Input: part model. Units: mm. Frame: model coordinates. Give positions to 0.01 mm unless a question says otherwise; leave off trailing zeros. Write each loop counter-clockwise with the first axis right and the second up, starting at its lowest first coordinate (ties: lowest second). Pieces come first, ordered by that corner, then holes. Notation, with made-up numbers: (-31.5, 4) -> (-10.5, 4) arc R17 cw to (-10.5, 15) -> close; hole circle Ø10 at (73, -31.75). An arc over 180 degrees is marked (long way). Return JSON: item names as keys, results as strings. Group by question number.
Item 1: Section C-C, the plane z = 5. Count the separate pieces of the cut face and the enclosed holes in it, then the cut area to 3 significant figures.
Item 2: Section A-A, the plane y = 0. Return loops of the section in (x, z), then the cut area to 3 significant figures.
Item 3: Mould query, pull axis X, two halves, no side actions, for faces 1 (the face through (-10, 24, 10)), 2 (the face through (11.515, -26.773, 5.07)), 3 (the face through (24.326, 24.816, 4.93)). Classes: released by +X, released by -X, zero draft, split by the parting line, or undercut.
Item 4: Section D-D, the plane x = -35. Return loops of the section in (y, z), then the cut area to 3 significant figures.
Item 5: Line query: line 1 (Y direction, x = 0, z = 5.25); line 2 (Y direction, x = -9, z = 3); line 3 (Y direction, x = 31, z = 4). Output: solid intervals per line, ascending. Write a range as [from, to].
Item 6: Pin query (flat end, axial travel): P1, Ø1, axis at x = -6, z = 6, coming from the +Y side; P2, Ø1, axis at x = -12, z = 7, coming from the +Y side; P3, Ø1.5, axis at x = 31, z = 8, coming from the +Y side. Return the tip coordinate at first contact, or that it passes through.
from build123d import *

# Parameters (mm, degrees)
SZKIC1_R                        = 5
SZKIC1_R_2                      = 25
DODANIE_WYCI_GNI_CIE1_DEPTH     = 10
WYTNIJ_WYCI_GNI_CIE1_DEPTH      = 65.420493634
WYTNIJ_WYCI_GNI_CIE1_DEPTH_BACK = 65.420493634
SZKIC2_R                        = 2.75


with BuildPart() as part:
    # Szkic1 → Dodanie-wyciągnięcie1 (new body)
    with BuildSketch(Plane.XY):
        with BuildLine():
            Line((-42.071067812, 7.071067812), (-7.071067812, 42.071067812))
            ThreePointArc((-7.071067812, 42.071067812), (0, 45), (7.071067812, 42.071067812))
            Line((7.071067812, 42.071067812), (42.071067812, 7.071067812))
            ThreePointArc((42.071067812, 7.071067812), (45, 0), (42.071067812, -7.071067812))
            Line((42.071067812, -7.071067812), (7.071067812, -42.071067812))
            ThreePointArc((7.071067812, -42.071067812), (0, -45), (-7.071067812, -42.071067812))
            Line((-7.071067812, -42.071067812), (-42.071067812, -7.071067812))
            ThreePointArc((-42.071067812, -7.071067812), (-45, 0), (-42.071067812, 7.071067812))
        make_face()
        with Locations((-35, 0)):
            Circle(SZKIC1_R, mode=Mode.SUBTRACT)
        with Locations((0, 35)):
            Circle(SZKIC1_R, mode=Mode.SUBTRACT)
        with Locations((35, 0)):
            Circle(SZKIC1_R, mode=Mode.SUBTRACT)
        with Locations((0, -35)):
            Circle(SZKIC1_R, mode=Mode.SUBTRACT)
        Circle(SZKIC1_R_2, mode=Mode.SUBTRACT)
    extrude(amount=DODANIE_WYCI_GNI_CIE1_DEPTH)

    # Szkic2 → Wytnij-wyciągnięcie1 (cut, two sides: drawn at the far end of the back side and taken through both)
    with BuildSketch(Plane(origin=(0, 0, 0), x_dir=(-1, 0, 0), z_dir=(0, 0, -1)).offset(-WYTNIJ_WYCI_GNI_CIE1_DEPTH_BACK)):
        with Locations((11.156854249, -29.5)):
            Circle(SZKIC2_R)
        with Locations((29.18807717, -11.46877708)):
            Circle(SZKIC2_R)
        with Locations((-11.156854249, -29.5)):
            Circle(SZKIC2_R)
        with Locations((-29.18807717, -11.46877708)):
            Circle(SZKIC2_R)
    extrude(amount=WYTNIJ_WYCI_GNI_CIE1_DEPTH + WYTNIJ_WYCI_GNI_CIE1_DEPTH_BACK, mode=Mode.SUBTRACT)


solid = part.part
Answer below:
{
 "1": {"separate pieces": "1", "enclosed holes": "9", "area": "2,370 mm2"},
 "2": {"outline": "(-45, 0) -> (-40, 0) -> (-40, 10) -> (-45, 10) -> close; (-30, 0) -> (-25, 0) -> (-25, 10) -> (-30, 10) -> close; (25, 0) -> (30, 0) -> (30, 10) -> (25, 10) -> close; (40, 0) -> (45, 0) -> (45, 10) -> (40, 10) -> close", "area": "200 mm2"},
 "3": {"face 1": "zero draft", "face 2": "undercut", "face 3": "released by +X"},
 "4": {"outline": "(-14.14, 0) -> (-5, 0) -> (-5, 10) -> (-14.14, 10) -> close; (5, 0) -> (14.14, 0) -> (14.14, 10) -> (5, 10) -> close", "area": "183 mm2"},
 "5": {"line 1": "y = [-45, -40], [-30, -25], [25, 30], [40, 45]", "line 2": "y = [-40.14, -31.21], [-27.79, -23.32], [23.32, 40.14]", "line 3": "y = [-18.14, -13.54], [-9.4, -3], [3, 18.14]"},
 "6": {"P1": "stops at y = 43.35", "P2": "stops at y = 37.64", "P3": "stops at y = 18.89"}
}
